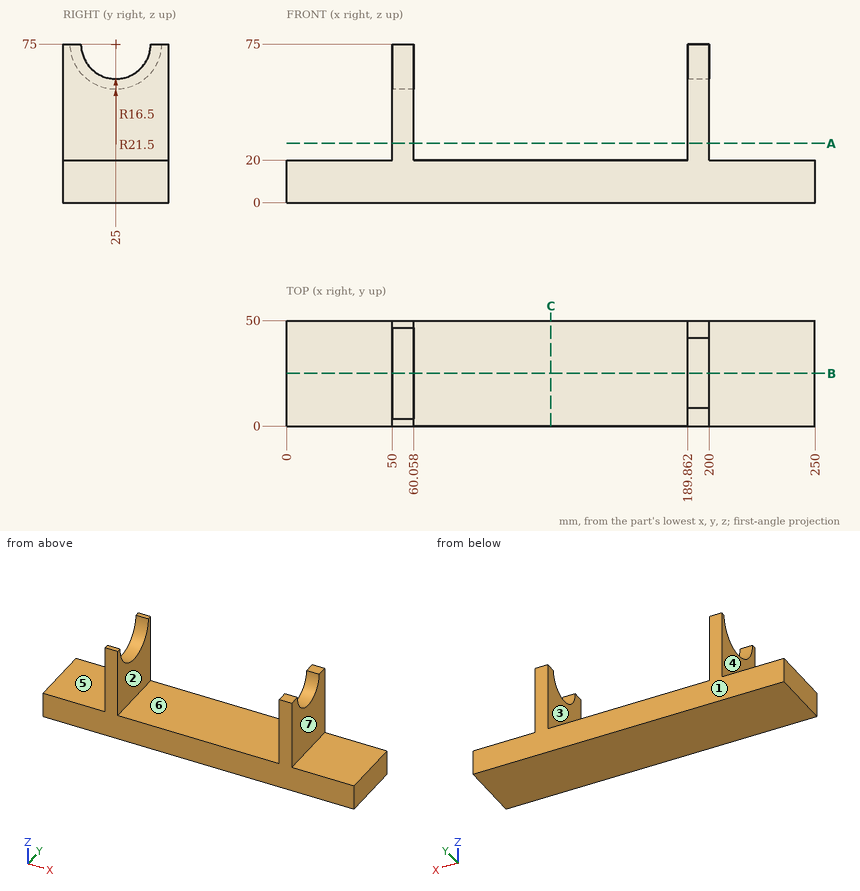
Drawing for the job (mm, zero at the part's lowest x, y, z). A direction names the side the tool comes from. Give positions to 0.01 mm unless a question says otherwise; leave off trailing zeros. Order: outer loops, then holes, each group sorted by start corner. A loop starts at its lowest first (then second) coordinate and runs counter-clockwise, first axis right, second up. Notation, with made-up numbers: M 3,-26.75 L 21,-26.75 A21 cw 21,3.25 Z; hole C 39,16.5 d5. An arc over 180 degrees is marked long. Write item = value, one per line. Start each with the question number.
(1) Slice it at B-B on y = 25. Write the cut outline in (x, z), plus the area to 3 significant figures.
(2) Slice it at A-A on z = 28. Write the cut outline in (x, y).
(3) Pin check, flat tips, straight feed: pin 1 Ø15 at (x, y) = (155.5, 21) entering from +Z; pin 2 Ø15 at (y, z) = (30.5, 48) entering from -X; pin 3 Ø8 at (y, z) = (31.5, 42.5) entering from +X. Stop position of each tip, or through.
(4) Two-plate mould, pull along X, no slides. Class the marked faces 1, 2, 3 and 4: released by +X, released by -X, zero draft, split by the parting line, or undercut.
(5) Probe L1, parallel to X at y = 10, z = 37; L2, parallel to Z at x = 112.5, y = 27; L3, parallel to X at y = 9, z = 63. List the from-to ranges inside material, lowest first. Write a range as [from, to].
(6) Slice it at C-C on x = 125. Write the cut outline in (y, z).
(7) Which spindle directions (+Z, -Z, +X, -X, +Y, -Y) get a long thin tool onto all of the face, cutting with end or side? Do the marked faces 5, 6 and 7. Say none if no direction does.
Responses:
q1.outline = M 0,0 L 250,0 L 250,20 L 200,20 L 200,58.5 L 189.86,58.5 L 189.86,20 L 60.06,20 L 60.06,53.5 L 50,53.5 L 50,20 L 0,20 Z
q1.area = 5,730 mm2
q2.outline = M 50,0 L 60.06,0 L 60.06,50 L 50,50 Z; M 189.86,0 L 200,0 L 200,50 L 189.86,50 Z
q3.pin_1 = 20
q3.pin_2 = 50
q3.pin_3 = 200
q4.face_1 = zero draft
q4.face_2 = undercut
q4.face_3 = undercut
q4.face_4 = released by -X
q5.L1 = [50, 60.06], [189.86, 200]
q5.L2 = [0, 20]
q5.L3 = [189.86, 200]
q6.outline = M 0,0 L 50,0 L 50,20 L 0,20 Z
q7.face_5 = +Z, -X, +Y, -Y
q7.face_6 = +Z, +Y, -Y
q7.face_7 = +Z, +X, +Y, -Y
